Autodesk Inventor part; units mm, degrees
ref_plane "YZ Plane" through (0, 0, 0) normal (1, 0, 0) x (0, 1, 0)
ref_plane "XZ Plane" through (0, 0, 0) normal (0, 1, 0) x (-1, 0, 0)
ref_plane "XY Plane" through (0, 0, 0) normal (0, 0, 1) x (1, 0, 0)
sketch "Sketch1" plane through (0, 0, 0) normal (0, 1, 0) x (-1, 0, 0)
  circle A0 centre (0, 0) radius 50
  circle A1 centre (0, 0) radius 15
  circle A2 centre (0, 0) radius 35 construction
  circle A3 centre (0, -35) radius 6
  circle A4 centre (30.3109, -17.5) radius 6
  circle A5 centre (30.3109, 17.5) radius 6
  circle A6 centre (0, 35) radius 6
  circle A7 centre (-30.3109, 17.5) radius 6
  circle A8 centre (-30.3109, -17.5) radius 6
  dimension "d2" = 70
  dimension "d0" = 100
  dimension "d1" = 30
  dimension "d3" = 12
  dimension "d6" = 360
extrude "Extrusion1" add sketch "Sketch1" along normal blind 15
sketch "Sketch2" plane through (0, 15, 0) normal (0, 1, 0) x (1, 0, 0)
  circle A0 centre (0, 0) radius 25
  circle A1 centre (0, 0) radius 15
  dimension "d10" = 50
extrude "Extrusion2" add sketch "Sketch2" along normal blind 70
sketch "Sketch3" plane through (0, 85, 0) normal (0, 1, 0) x (1, 0, 0)
  circle A0 centre (-50, 0) radius 13
  circle A1 centre (-50, 0) radius 5
  circle A2 centre (50, 0) radius 13
  circle A3 centre (50, 0) radius 5
  circle A4 centre (0, 0) radius 50 construction
  circle A5 centre (0, 0) radius 25
  circle A6 centre (0, 0) radius 15
  line L0 (-6, 24.2693) -> (-53.12, 12.62)
  line L1 (-6, -24.2693) -> (-53.12, -12.62)
  line L2 (6, 24.2693) -> (53.12, 12.62)
  line L3 (6, -24.2693) -> (53.12, -12.62)
  dimension "d13" = 26
  dimension "d14" = 10
  dimension "d15" = 26
  dimension "d16" = 10
  dimension "d17" = 100
extrude "Extrusion3" add sketch "Sketch3" along normal blind 15
properties part number "Exercise05"
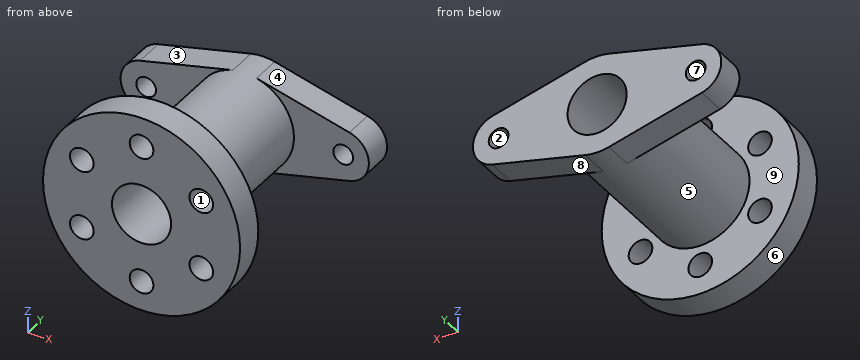
Geometry: final body of the model. Coordinates: model frame, mm. Face numbers are marked on the shaded views. A direction names the side the tool comes from. Round coordinates to 2 decimals unless told otherwise and drop trailing zeros. Order: outer loops, then holes, each group sorted by start corner. A loop starts at its lowest first (then second) coordinate and runs counter-clockwise, first axis right, second up. Notation, with made-up numbers: M 26.5,72.25 L 66.5,72.25 A22 ccw 66.5,100.25 Z; hole C 9,10.5 d3. An arc over 180 degrees is marked long. One line per item, written item: value.
(1) Pin query (flat end, axial travel): P1, Ø4, axis at y = 59.5, z = 7.5, coming from the -X side; P2, Ø2, axis at x = -12, z = 28.5, coming from the -Y side; P3, Ø8, axis at x = -3.5, z = -34, coming from the +Y side; P4, Ø7, axis at x = -30.31, z = 17.5, coming from the -Y side. Return the tip coordinate at first contact, or that it passes through.
Result sheet:
P1: x = -24.39
P2: y = 0
P3: y = 15
P4: y = 85
(2) Cut plane C-C (x = -40). Return the cut outline in (y, z), and give its area (3 significant figures).
Result sheet:
outline: M 0,-30 L 15,-30 L 15,30 L 0,30 Z; M 85,-15.86 L 100,-15.86 L 100,15.86 L 85,15.86 Z
area: 1,380 mm2
(3) Line query: probe 1 along Z at (x, y) = (0, 11); probe 2 along X at (y, z) = (7, -17); probe 3 along Y at (x, z) = (9.5, -36.5). Output: solid intervals per line, ascending. Write a range as [from, to].
Result sheet:
probe 1: [-50, -41], [-29, -15], [15, 29], [41, 50]
probe 2: [-47.02, -36.29], [-24.33, 24.33], [36.29, 47.02]
probe 3: [0, 15]
(4) Cut plane B-B (z = -2). Return the cut outline in (x, y), and give its area (3 significant figures).
Result sheet:
outline: M -62.85,85 L -54.58,85 L -54.58,100 L -62.85,100 Z; M -49.96,0 L -14.87,0 L -14.87,100 L -45.42,100 L -45.42,85 L -24.92,85 L -24.92,15 L -49.96,15 Z; M 14.87,0 L 49.96,0 L 49.96,15 L 24.92,15 L 24.92,85 L 45.42,85 L 45.42,100 L 14.87,100 Z; M 54.58,85 L 62.85,85 L 62.85,100 L 54.58,100 Z
area: 3,620 mm2
(5) Pull-direction query (X, two-part tool) for the marked faces 6, 7, 8 and 9; classes: pulls with the +X half, pulls with the -X half, needs draft (parallel to the pull), parting line crosses it, or undercut.
Result sheet:
face 6: parting line crosses it
face 7: undercut
face 8: pulls with the +X half
face 9: needs draft
(6) Cut plane D-D (z = -33). Return the cut outline in (x, y), and give its area (3 significant figures).
Result sheet:
outline: M -37.56,0 L -5.66,0 L -5.66,15 L -37.56,15 Z; M 5.66,0 L 37.56,0 L 37.56,15 L 5.66,15 Z
area: 957 mm2
(7) Cut plane A-A (y = 6.5). Return the cut outline in (x, z), and give its area (3 significant figures).
Result sheet:
outline: C 0,0 d100; hole C -30.31,-17.5 d12; hole C -30.31,17.5 d12; hole C 0,0 d30; hole C 0,-35 d12; hole C 0,35 d12; hole C 30.31,-17.5 d12; hole C 30.31,17.5 d12
area: 6,470 mm2
(8) Reachability of the marked faces 1, 2, 3, 4 and 5 from +Z, -Z, +X, -X, +Y, -Y: full face, straight path, thin tool, end or side. Return the list, or none.
Result sheet:
face 1: -Y
face 2: +Y
face 3: +Z, -X, +Y
face 4: +Z, +X, +Y
face 5: none
